Input: part model. Units: mm. Frame: model coordinates. A direction names the side the tool comes from. Round coordinates to 2 decimals unless told otherwise and drop trailing zeros. Order: outer loops, then holes, each group sorted by start corner. A loop starts at its lowest first (then second) coordinate and runs counter-clockwise, first axis right, second up. Notation, with made-up numbers: (-24, -22) -> (-1, -22) arc R25 ccw to (-1, 8) -> close; hole circle Ø1 at (15.25, 52.5). An arc over 180 degrees is marked (long way). Use a Markdown table: item, result.
from build123d import *

# Parameters (mm, degrees)
BOSS_EXTRUDE1_DEPTH = 15
SKETCH2_R           = 6
BOSS_EXTRUDE2_DEPTH = 5
SKETCH2_2_R         = 6
BOSS_EXTRUDE3_DEPTH = 1
BOSS_EXTRUDE4_START = 1
SKETCH3_W           = 0.5
SKETCH3_H           = 4.5
BOSS_EXTRUDE4_DEPTH = 2.5
FILLET1_R           = 1.5
FILLET2_R           = 1.5


with BuildPart() as part:
    # Sketch1 → Boss-Extrude1 (new body)
    with BuildSketch(Plane(origin=(0, 0, 0), x_dir=(1, 0, 0), z_dir=(0, 1, 0))):
        with BuildLine():
            Line((-2.375, 10), (2.375, 10))
            Line((2.375, 10), (2.375, 3.218598297))
            ThreePointArc((2.375, 3.218598297), (2.828427125, 2.828427125), (3.218598297, 2.375))
            Line((3.218598297, 2.375), (10, 2.375))
            Line((10, 2.375), (10, -2.375))
            Line((10, -2.375), (3.218598297, -2.375))
            ThreePointArc((3.218598297, -2.375), (2.828427125, -2.828427125), (2.375, -3.218598297))
            Line((2.375, -3.218598297), (2.375, -10))
            Line((2.375, -10), (-2.375, -10))
            Line((-2.375, -10), (-2.375, -3.218598297))
            ThreePointArc((-2.375, -3.218598297), (-2.828427125, -2.828427125), (-3.218598297, -2.375))
            Line((-3.218598297, -2.375), (-10, -2.375))
            Line((-10, -2.375), (-10, 2.375))
            Line((-10, 2.375), (-3.218598297, 2.375))
            ThreePointArc((-3.218598297, 2.375), (-2.828427125, 2.828427125), (-2.375, 3.218598297))
            Line((-2.375, 3.218598297), (-2.375, 10))
        make_face()
    extrude(amount=-BOSS_EXTRUDE1_DEPTH)


with BuildPart() as body_2:
    # Sketch2 → Boss-Extrude2 (new body)
    with BuildSketch(Plane(origin=(0, 0, 0), x_dir=(1, 0, 0), z_dir=(0, 1, 0))):
        with Locations(Location((0, 0, 0), (0, 0, 270))):
            Circle(SKETCH2_R)
    extrude(amount=-BOSS_EXTRUDE2_DEPTH)

    # Sketch2<2> → Boss-Extrude3 (add)
    with BuildSketch(Plane(origin=(0, 0, 0), x_dir=(1, 0, 0), z_dir=(0, 1, 0))):
        with Locations(Location((0, 0, 0), (0, 0, 270))):
            Circle(SKETCH2_2_R)
    extrude(amount=BOSS_EXTRUDE3_DEPTH)

    # Combine1: cut part
    add(part.part, mode=Mode.SUBTRACT)

    # Sketch3 → Boss-Extrude4 (add)
    with BuildSketch(Plane(origin=(0, 0, 0), x_dir=(1, 0, 0), z_dir=(0, 1, 0)).offset(BOSS_EXTRUDE4_START)):
        Rectangle(SKETCH3_W, SKETCH3_H)
    extrude(amount=BOSS_EXTRUDE4_DEPTH)

    # Fillet1
    fillet1_edges = [body_2.edges().sort_by_distance(p)[0] for p in [
        (0.25, 1, 0),
        (-0.25, 1, 0),
    ]]
    fillet(fillet1_edges, radius=FILLET1_R)

    # Fillet2
    fillet2_edges = [body_2.edges().sort_by_distance(p)[0] for p in [
        (0, 1, -2.25),
        (0, 1, 2.25),
    ]]
    fillet(fillet2_edges, radius=FILLET2_R)

    # Sketch4 → Revolve1 (revolve)
    with BuildSketch(Plane(origin=(0, 0, 0), x_dir=(0, 0, -1), z_dir=(1, 0, 0)), mode=Mode.PRIVATE) as revolve1_sk:
        Polygon((-6, 1), (-6, 4), (-5, 4), (-4.2, 1), align=None)
    revolve(revolve1_sk.sketch.rotate(Axis((0, 0, 0), (0, 1, 0)), 180), axis=Axis((0, 0, 0), (0, 1, 0)))

    # Fillet3: read off the stored shape, not the designer's step
    # Fillet3 outline → Fillet3 (revolve)
    with BuildSketch(Plane.XY):
        with BuildLine():
            ThreePointArc((4.34846747, 1.556753012), (4.08071837, 1.155258358), (3.623791265, 1))
            Line((3.623791265, 1), (4.34846747, 1))
            Line((4.34846747, 1), (4.34846747, 1.556753012))
        make_face()
    revolve(axis=Axis((0, 0, 0), (0, 1, 0)))


solid = body_2.part
1) Cut plane A-A on y = -2.25. Return loops of the section in (x, z) (3 decimals).
Answer key:
| item | result |
|---|---|
| outline | (-5.51, -2.375) arc R6 ccw to (-2.375, -5.51) -> (-2.375, -3.219) arc R4 cw to (-3.219, -2.375) -> close; (-5.51, 2.375) -> (-3.219, 2.375) arc R4 cw to (-2.375, 3.219) -> (-2.375, 5.51) arc R6 ccw to start; (2.375, -5.51) arc R6 ccw to (5.51, -2.375) -> (3.219, -2.375) arc R4 cw to (2.375, -3.219) -> close; (2.375, 3.219) arc R4 cw to (3.219, 2.375) -> (5.51, 2.375) arc R6 ccw to (2.375, 5.51) -> close |
2) Draft query along X for faces 1 (the face through (4, -2, -2.375)), 2 (the face through (-0.021, 1.288, 2.866)). Return one class per face: released by +X, released by -X, zero draft, split by the parting line, or undercut.
Answer key:
| item | result |
|---|---|
| face 1 | zero draft |
| face 2 | undercut |
3) Contact query for flat-ended pins moving along their axis: P1, Ø0.7, axis at x = -4.5, y = -2.5, coming from the +Z side; P2, Ø1, axis at y = -4, z = -4.5, coming from the -X side; P3, Ø1.8, axis at y = -3.5, z = 4, coming from the +X side; P4, Ø1, axis at x = 1.5, y = -3.5, coming from the -Z side. Output: stop coordinate, or through.
Answer key:
| item | result |
|---|---|
| P1 | stops at z = 4.33 |
| P2 | stops at x = -4.47 |
| P3 | stops at x = 5.14 |
| P4 | passes through |
4) Cut plane D-D on z = 0. Return loops of the section in (x, y).
Answer key:
| item | result |
|---|---|
| outline | (-6, 0) -> (6, 0) -> (6, 4) -> (5, 4) -> (4.35, 1.56) arc R0.75 cw to (3.62, 1) -> (1.75, 1) arc R1.5 cw to (0.25, 2.5) -> (0.25, 3.5) -> (-0.25, 3.5) -> (-0.25, 2.5) arc R1.5 cw to (-1.75, 1) -> (-3.62, 1) arc R0.75 cw to (-4.35, 1.56) -> (-5, 4) -> (-6, 4) -> close |
5) Set-up query: faces 3 (the face through (-2, 1, 0)), 4 (the face through (-4, -2, -2.375)), 5 (the face through (2.822, -2.465, -2.834)). Return all of +Z, -Z, +X, -X, +Y, -Y with unobstructed straight access to the full face (end or side cutting, diameter ignored); none if empty.
Answer key:
| item | result |
|---|---|
| face 3 | +Y |
| face 4 | +X, -X, -Y |
| face 5 | -Y |
6) Cut plane C-C on x = 0. Return loops of the section in (y, z).
Answer key:
| item | result |
|---|---|
| outline | (0, -6) -> (4, -6) -> (4, -5) -> (1.56, -4.35) arc R0.75 cw to (1, -3.68) arc R1.5 cw to (2.5, -2.25) -> (3.5, -2.25) -> (3.5, 2.25) -> (2.5, 2.25) arc R1.5 cw to (1, 3.68) arc R0.75 cw to (1.56, 4.35) -> (4, 5) -> (4, 6) -> (0, 6) -> close |
7) Cut plane B-B on y = 1.75. Return loops of the section in (x, z).
Answer key:
| item | result |
|---|---|
| outline | circle Ø12 at (0, 0); (-0.45, -2.45) -> (0.45, -2.45) -> (0.45, 2.45) -> (-0.45, 2.45) -> close; hole circle Ø8.8 at (0, 0) |
8) Ray query, probe 1 along X at (y, z) = (3, 0); probe 2 along Z at (x, y) = (-0.5, 2.5); probe 3 along X at (y, z) = (1.5, -4). Return the intervals inside material, ascending.
Answer key:
| item | result |
|---|---|
| probe 1 | x = -6 to -4.73, -0.25 to 0.25, 4.73 to 6 |
| probe 2 | z = -5.98 to -4.57, 4.57 to 5.98 |
| probe 3 | x = -4.47 to -1.66, 1.66 to 4.47 |
